Check sheet for the modelled part. Datum: model origin and axes. Units: mm. A direction names the side the tool comes from. Round coordinates to 2 decimals unless told otherwise and drop trailing zeros. Loops run counter-clockwise (first coordinate to the right, second up) from the corner with the lowest first, then second, coordinate; pieces in that order, holes last. Notation, with made-up numbers: (51, -14) -> (63, -14) arc R20 cw to (63, 8) -> close; hole circle Ø7 at (87, -9.5). An arc over 180 degrees is marked (long way). One line per question, with ' | ' between items.
```python
from build123d import *

# Parameters (mm, degrees)
SKETCH2_W           = 40
SKETCH2_H           = 200
BOSS_EXTRUDE1_DEPTH = 30
SKETCH3_R           = 2
CUT_EXTRUDE1_DEPTH  = 10
FILLET1_R           = 20
SKETCH5_R           = 7.5
CUT_EXTRUDE3_DEPTH  = 20
FILLET2_R           = 18
SKETCH6_W           = 10
SKETCH6_H           = 150
CUT_EXTRUDE4_DEPTH  = 112.803398875
SKETCH7_W           = 5
SKETCH7_H           = 10
BOSS_EXTRUDE2_DEPTH = 15


with BuildPart() as part:
    # Sketch2 → Boss-Extrude1 (new body)
    with BuildSketch(Plane.XY):
        Rectangle(SKETCH2_W, SKETCH2_H)
    extrude(amount=BOSS_EXTRUDE1_DEPTH)

    # Sketch3 → Cut-Extrude1 (cut)
    with BuildSketch(Plane(origin=(0, 0, 0), x_dir=(-1, 0, 0), z_dir=(0, 0, -1))):
        with Locations((0, -90)):
            Circle(SKETCH3_R)
    extrude(amount=-CUT_EXTRUDE1_DEPTH, mode=Mode.SUBTRACT)

    # Fillet1
    fillet1_edges = [part.edges().sort_by_distance(p)[0] for p in [
        (20, -100, 15),
        (-20, -100, 15),
    ]]
    fillet(fillet1_edges, radius=FILLET1_R - 0.0001)  # a hair under: the kernel refuses the full size

    # Sketch5 → Cut-Extrude3 (cut)
    with BuildSketch(Plane.XY.offset(30)):
        with Locations((0, 88)):
            Circle(SKETCH5_R)
    extrude(amount=-CUT_EXTRUDE3_DEPTH, mode=Mode.SUBTRACT)

    # Fillet2
    fillet2_edges = [part.edges().sort_by_distance(p)[0] for p in [
        (-20, 100, 15),
        (20, 100, 15),
    ]]
    fillet(fillet2_edges, radius=FILLET2_R)

    # Sketch6 → Cut-Extrude4 (cut, through all)
    with BuildSketch(Plane.ZY.offset(20)):
        with Locations((15, -5)):
            Rectangle(SKETCH6_W, SKETCH6_H)
    extrude(amount=-CUT_EXTRUDE4_DEPTH, mode=Mode.SUBTRACT)

    # Sketch7 → Boss-Extrude2 (add)
    with BuildSketch(Plane(origin=(0, 0, 20), x_dir=(-1, 0, 0), z_dir=(0, 0, -1))):
        with Locations((17.5, -10)):
            Rectangle(SKETCH7_W, SKETCH7_H)
    boss_extrude2 = extrude(amount=BOSS_EXTRUDE2_DEPTH)

    # Mirror1: Boss-Extrude2 across plane
    add(boss_extrude2.mirror(Plane(origin=(0, 0, 0), x_dir=(0, 0, 1), z_dir=(1, 0, 0))))


solid = part.part
```
(1) Sectioned sample at A-A, the plane z = 16. Count the separate pieces of the cut face and the enclosed holes in it, and give its area (3 significant figures).
Answer:
separate pieces: 4 | enclosed holes: 1 | area: 1,610 mm2
(2) Sectioned sample at D-D, the plane x = -12.5. Record the cut outline in (y, z), and give its area (3 significant figures).
Answer:
outline: (-95.61, 0) -> (96.62, 0) -> (96.62, 30) -> (-95.61, 30) -> close; hole (-80, 10) -> (70, 10) -> (70, 20) -> (-80, 20) -> close | area: 4,270 mm2
(3) Set-up check for faces 4 (the face through (0, -90, 10)), 5 (the face through (-14.867, 94.587, 15.21)), 6 (the face through (15, -10, 15)), 7 (the face through (-17, -5, 15)), 8 (the face through (-1.63, 80.68, 20.14)): record each of +Z, -Z, +X, -X, +Y, -Y from which the full face is reachable in a straight line by a thin tool's end or side.
Answer:
face 4: -Z | face 5: +Z, -Z, -X, +Y | face 6: none | face 7: +X, -X | face 8: +Z
(4) Go/stop test with flat-tipped pins: pin 1 (1 mm diameter, centred on x = -8.5, z = 9.5, fed in from -Y); pin 2 (1.5 mm diameter, centred on x = 17.5, z = 17.5, fed in from +Y); pin 3 (5 mm diameter, centred on x = 12.5, z = 5.5, fed in from +Y). Record where each tip stops, or that it passes through.
Answer:
pin 1: stops at y = -98.33 | pin 2: stops at y = 92.32 | pin 3: stops at y = 98.12
(5) Mould release check, pull along Z, two halves, no side actions. Record for faces 1 (the face through (0, -80, 15)), 2 (the face through (0, 88, 10)), 3 (the face through (0, 100, 15)): +Z half, -Z half, draft (parallel to the pull), parting line (faces both ways), or undercut.
Answer:
face 1: undercut | face 2: +Z half | face 3: draft
(6) Scan lines: probe 1 along Z at (x, y) = (-17.5, 47); probe 2 along Y at (x, z) = (0, 7.75); probe 3 along Y at (x, z) = (0.5, 22.5). Record each from-to range of solid material in increasing order.
Answer:
probe 1: z = 0 to 10, 20 to 30 | probe 2: y = -100 to -92, -88 to 100 | probe 3: y = -99.99 to 80.52, 95.48 to 100
(7) Sectioned sample at B-B, the plane y = -72. Record the cut outline in (x, z), and give its area (3 significant figures).
Answer:
outline: (-20, 0) -> (20, 0) -> (20, 10) -> (-20, 10) -> close; (-20, 20) -> (20, 20) -> (20, 30) -> (-20, 30) -> close | area: 800 mm2
